```python
from build123d import *

# Parameters (mm, degrees)
SKETCH_R      = 19
SKETCH_R_2    = 12
PAD_DEPTH     = 1
SKETCH001_R   = 15.95
SKETCH001_R_2 = 13.95
PAD001_DEPTH  = 20
SKETCH002_R   = 13.95
SKETCH002_R_2 = 12
PAD002_DEPTH  = 3


with BuildPart() as part:
    # Sketch → Pad (new body)
    with BuildSketch(Plane.XY):
        Circle(SKETCH_R)
        Circle(SKETCH_R_2, mode=Mode.SUBTRACT)
    extrude(amount=PAD_DEPTH)

    # Sketch001 → Pad001 (new body)
    with BuildSketch(Plane.XY.offset(1)):
        Circle(SKETCH001_R)
        Circle(SKETCH001_R_2, mode=Mode.SUBTRACT)
    extrude(amount=PAD001_DEPTH)

    # Sketch002 → Pad002 (new body)
    with BuildSketch(Plane.XY.offset(1)):
        Circle(SKETCH002_R)
        Circle(SKETCH002_R_2, mode=Mode.SUBTRACT)
    extrude(amount=PAD002_DEPTH)


solid = part.part
```
Build history of the part. All positions in model axes, mm. A direction names the side the tool comes from. Coordinates: 2 decimals unless noted, no trailing zeros. Order: outer loops, then holes, each group sorted by start corner. A loop starts at its lowest first (then second) coordinate and runs counter-clockwise, first axis right, second up. Notation, with made-up numbers: M -25,9 L 28,9 A19 ccw 28,31 Z; hole C 26,56 d10. An arc over 180 degrees is marked long. One line per question, with ' | ' between items. Start each with the question number.
1. Cut at A-A (y = 0). Write the cut outline in (x, z), plus the area to 3 significant figures.
2. Wall check: line 1 along Y through (x, z) = (0, 2.25); line 2 along X through (y, z) = (7, 1.5); line 3 along Z through (x, y) = (13, 4). Give the ranges that are in metal, low to high. Write a range as [from, to].
3. Cut at C-C (z = 2.75). Write the cut outline in (x, y).
4. Flat gauge pins, fed straight in: P1, Ø5, axis at y = -2, z = 4, coming from the +X side; P2, Ø4, axis at x = 5, z = 18, coming from the -Y side; P3, Ø1, axis at y = 12, z = 12, coming from the +X side. Where does each tip first touch, or does it go through?
5. Mould opens along Y. For faces 1 (the face through (15.213, 4.791, 10.86)), 2 (the face through (-0.1, -14.1, 21)), 3 (the face through (-11.99, 0.53, 1.97)) say: +Y half, -Y half, draft (parallel to the pull), parting line (faces both ways), or undercut.
6. Cut at D-D (z = 13.25). Write the cut outline in (x, y).
7. Tool access for faces 4 (the face through (8.767, -16.856, 0.493)), 5 (the face through (-3.02, -13.62, 12.38)): list every direction of +Z, -Z, +X, -X, +Y, -Y with a clear straight run to the whole face (end or side of a thin tool).
The answers:
1) outline: M -19,0 L -12,0 L -12,4 L -13.95,4 L -13.95,21 L -15.95,21 L -15.95,1 L -19,1 Z; M 12,0 L 19,0 L 19,1 L 15.95,1 L 15.95,21 L 13.95,21 L 13.95,4 L 12,4 Z | area: 106 mm2
2) line 1: y = [-15.95, -12], [12, 15.95] | line 2: x = [-14.33, -9.75], [9.75, 14.33] | line 3: z = [0, 4]
3) outline: C 0,0 d31.9; hole C 0,0 d24
4) P1: stops at x = 15.95 | P2: stops at y = -15.67 | P3: stops at x = 11.05
5) face 1: parting line | face 2: draft | face 3: undercut
6) outline: C 0,0 d31.9; hole C 0,0 d27.9
7) face 4: +Z, -Z | face 5: +Z
